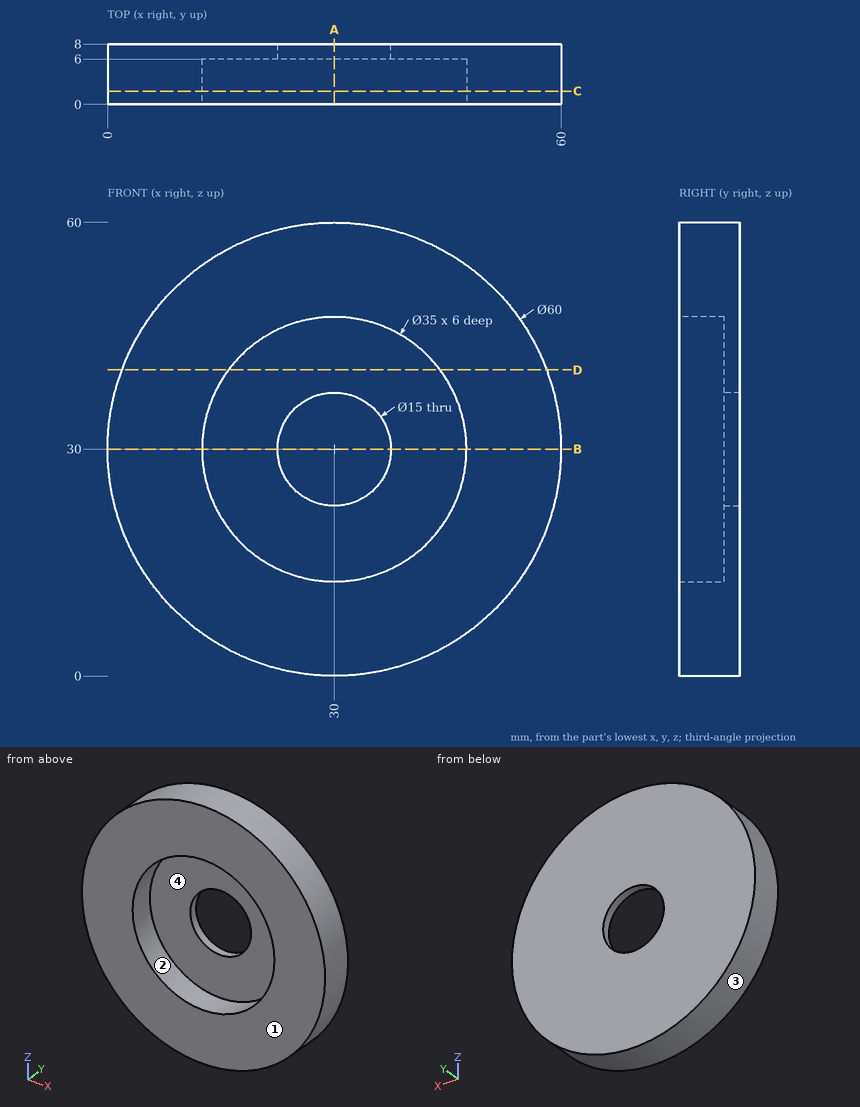
Part print with two shaded views. Sizes in mm from the minimum x, y, z corner. Coordinates: 2 decimals unless noted, no trailing zeros. Order: outer loops, then holes, each group sorted by start corner. A loop starts at its lowest first (then second) coordinate and runs counter-clockwise, first axis right, second up. Notation, with made-up numbers: (17.25, 34.5) - (75.25, 34.5) arc R6 cw to (75.25, 42.5) - close; hole circle Ø1 at (-33.75, 61.25). An arc over 180 degrees is marked (long way). Write item = value, one per line. Start each with the question number.
1) Saw through at A-A on x = 30. Write the cut outline in (y, z).
2) Flat gauge pins, fed straight in: pin 1 Ø1.5 at (x, y) = (41.5, 2.5) entering from -Z; pin 2 Ø10.5 at (x, z) = (27, 31) entering from -Y; pin 3 Ø3 at (x, y) = (27.5, 1) entering from -Z. Where does each tip first touch, or does it go through?
3) Two-plate mould, pull along Z, no slides. Class the marked faces 1, 2, 3 and 4: pulls with the +Z half, pulls with the -Z half, needs draft (parallel to the pull), parting line crosses it, or undercut.
4) Saw through at B-B on z = 30. Write the cut outline in (x, y), then the cut area to 3 significant figures.
5) Saw through at D-D on z = 40.5. Write the cut outline in (x, y).
6) Wall check: line 1 along X through (y, z) = (1.8, 30); line 2 along X through (y, z) = (7.3, 30); line 3 along Y through (x, z) = (13, 26). Give the ranges that are in metal, low to high. Write a range as from..to.
7) Saw through at C-C on y = 1.75. Write the cut outline in (x, z).
From the geometry:
q1.outline = (0, 0) - (8, 0) - (8, 22.5) - (6, 22.5) - (6, 12.5) - (0, 12.5) - close; (0, 47.5) - (6, 47.5) - (6, 37.5) - (8, 37.5) - (8, 60) - (0, 60) - close
q2.pin_1 = 1.99
q2.pin_2 = 6
q2.pin_3 = 0.02
q3.face_1 = needs draft
q3.face_2 = undercut
q3.face_3 = parting line crosses it
q3.face_4 = undercut
q4.outline = (0, 0) - (12.5, 0) - (12.5, 6) - (22.5, 6) - (22.5, 8) - (0, 8) - close; (37.5, 6) - (47.5, 6) - (47.5, 0) - (60, 0) - (60, 8) - (37.5, 8) - close
q4.area = 240 mm^2
q5.outline = (1.9, 0) - (16, 0) - (16, 6) - (44, 6) - (44, 0) - (58.1, 0) - (58.1, 8) - (1.9, 8) - close
q6.line_1 = 0..12.5, 47.5..60
q6.line_2 = 0..22.5, 37.5..60
q6.line_3 = 6..8
q7.outline = circle Ø60 at (30, 30); hole circle Ø35 at (30, 30)
